Can you work these out from the model? Positions are in its coordinate system, mm. A direction names the side the tool comes from. Round coordinates to 2 decimals unless told otherwise and drop trailing zeros. Loops run counter-clockwise (first coordinate to the right, second up) from the corner with the lowest first, then second, coordinate; pieces in that order, holes last. Notation, with made-up numbers: (53, 68.5) -> (62, 68.5) arc R31 cw to (62, 105.5) -> close; hole circle Ø2 at (31.5, 45). An arc over 180 degrees is marked (long way). Answer as a JSON object with one key per item and string values.
```python
from build123d import *

# Parameters (mm, degrees)
SKETCH_1_W          = 19.5
SKETCH_1_H          = 25
EXTRUDE_1_DEPTH     = 1
SKETCH_2_W          = 19.5
SKETCH_2_H          = 1
EXTRUDE_2_DEPTH     = 19.5
SKETCH_3_R          = 1.5
CUT_EXTRUDE_1_DEPTH = 26.130907266
SKETCH_4_R          = 4.25
CUT_EXTRUDE_2_DEPTH = 26.383311447


with BuildPart() as part:
    # 草图1 → 凸台-拉伸1 (new body)
    with BuildSketch(Plane.XY):
        Rectangle(SKETCH_1_W, SKETCH_1_H)
    extrude(amount=EXTRUDE_1_DEPTH)

    # 草图2 → 凸台-拉伸2 (add)
    with BuildSketch(Plane(origin=(0, 0, 0), x_dir=(-1, 0, 0), z_dir=(0, 0, -1))):
        Rectangle(SKETCH_2_W, SKETCH_2_H)
    extrude(amount=EXTRUDE_2_DEPTH)

    # 草图3 → 切除-拉伸1 (cut, through all)
    with BuildSketch(Plane(origin=(0, 0, 0), x_dir=(-1, 0, 0), z_dir=(0, 0, -1))):
        with Locations((5.100590272, 7.002287459)):
            Circle(SKETCH_3_R)
        with Locations(Location((-5.100590272, 7.002287459, 0), (0, 0, 180))):
            Circle(SKETCH_3_R)
        with Locations(Location((5.100590272, -7.002287459, 0), (0, 0, 180))):
            Circle(SKETCH_3_R)
        with Locations((-5.100590272, -7.002287459)):
            Circle(SKETCH_3_R)
    extrude(amount=-CUT_EXTRUDE_1_DEPTH, mode=Mode.SUBTRACT)

    # 草图4 → 切除-拉伸2 (cut, through all)
    with BuildSketch(Plane(origin=(0, 0.5, 0), x_dir=(1, 0, 0), z_dir=(0, 1, 0))):
        with Locations(Location((0, 9.75, 0), (0, 0, 180))):
            Circle(SKETCH_4_R)
    extrude(amount=-CUT_EXTRUDE_2_DEPTH, mode=Mode.SUBTRACT)


solid = part.part
```
Q1. I want a section at A-A, the plane z = -13.5. Write out the boundary of the cut face in (x, y).
Determined:
{"outline": "(-9.75, -0.5) -> (-2, -0.5) -> (-2, 0.5) -> (-9.75, 0.5) -> close; (2, -0.5) -> (9.75, -0.5) -> (9.75, 0.5) -> (2, 0.5) -> close"}
Q2. I want a section at C-C, the plane z = -1.5. Write out the boundary of the cut face in (x, y), then the cut area to 3 significant figures.
Determined:
{"outline": "(-9.75, -0.5) -> (9.75, -0.5) -> (9.75, 0.5) -> (-9.75, 0.5) -> close", "area": "19.5 mm²"}
Q3. On a 3-axis mill with a long thin cutter (end or side, diameter ignored), from which of +Z, -Z, +X, -X, +Y, -Y can I reach the whole of each face in a straight line? I mean faces 5 (the flat face through (0, 0, 1)), 6 (the flat face through (4.5, 0.5, -9.6)), 7 (the flat face through (0, -6, 0)). Say none if no direction works.
Determined:
{"face 5": "+Z, +X, -X, +Y, -Y", "face 6": "-Z, +X, -X, +Y", "face 7": "-Z, +X, -X, -Y"}
Q4. I'm going to push flat-ended pins straight in: pin 1 (2 mm diameter, centred on x = -7.5, z = -16.5, fed in from -Y); pin 2 (10 mm diameter, centred on x = 3.5, z = -14, fed in from +Y); pin 3 (5 mm diameter, centred on x = 5.1, y = -7, fed in from -Z). Where does each tip first touch, or does it pass through?
Determined:
{"pin 1": "y = -0.5", "pin 2": "y = 0.5", "pin 3": "z = 0"}
Q5. If I drill on L1, parallel to Z at x = 0, y = -0.2; L2, parallel to Z at x = 6, y = -9.25; L3, parallel to Y at x = 5, z = -16, over which ranges is the centre line in solid material (lowest first)? Write a range as [from, to].
Determined:
{"L1": "[-19.5, -14], [-5.5, 1]", "L2": "[0, 1]", "L3": "[-0.5, 0.5]"}
Q6. We'd pull the mould along Y, two halves only. Please class faces 1 (the cylindrical face through (-5.907, 8.267, 0.493)), 2 (the flat face through (-0.1, 12.5, 0.5)), 3 (the flat face through (0, 7, 0)), 4 (the cylindrical face through (-3.67, -7.45, 0.49)): pulls with the +Y half, pulls with the -Y half, needs draft (parallel to the pull), parting line crosses it, or undercut.
Determined:
{"face 1": "undercut", "face 2": "pulls with the +Y half", "face 3": "needs draft", "face 4": "undercut"}
Q7. I want a section at B-B, the plane x = 0. Write out the boundary of the cut face in (y, z), then the cut area to 3 significant figures.
Determined:
{"outline": "(-12.5, 0) -> (-0.5, 0) -> (-0.5, -5.5) -> (0.5, -5.5) -> (0.5, 0) -> (12.5, 0) -> (12.5, 1) -> (-12.5, 1) -> close; (-0.5, -19.5) -> (0.5, -19.5) -> (0.5, -14) -> (-0.5, -14) -> close", "area": "36.0 mm²"}
Q8. I want a section at D-D, the plane x = 2.75. Write out the boundary of the cut face in (y, z).
Determined:
{"outline": "(-12.5, 0) -> (-0.5, 0) -> (-0.5, -6.51) -> (0.5, -6.51) -> (0.5, 0) -> (12.5, 0) -> (12.5, 1) -> (-12.5, 1) -> close; (-0.5, -19.5) -> (0.5, -19.5) -> (0.5, -12.99) -> (-0.5, -12.99) -> close"}
